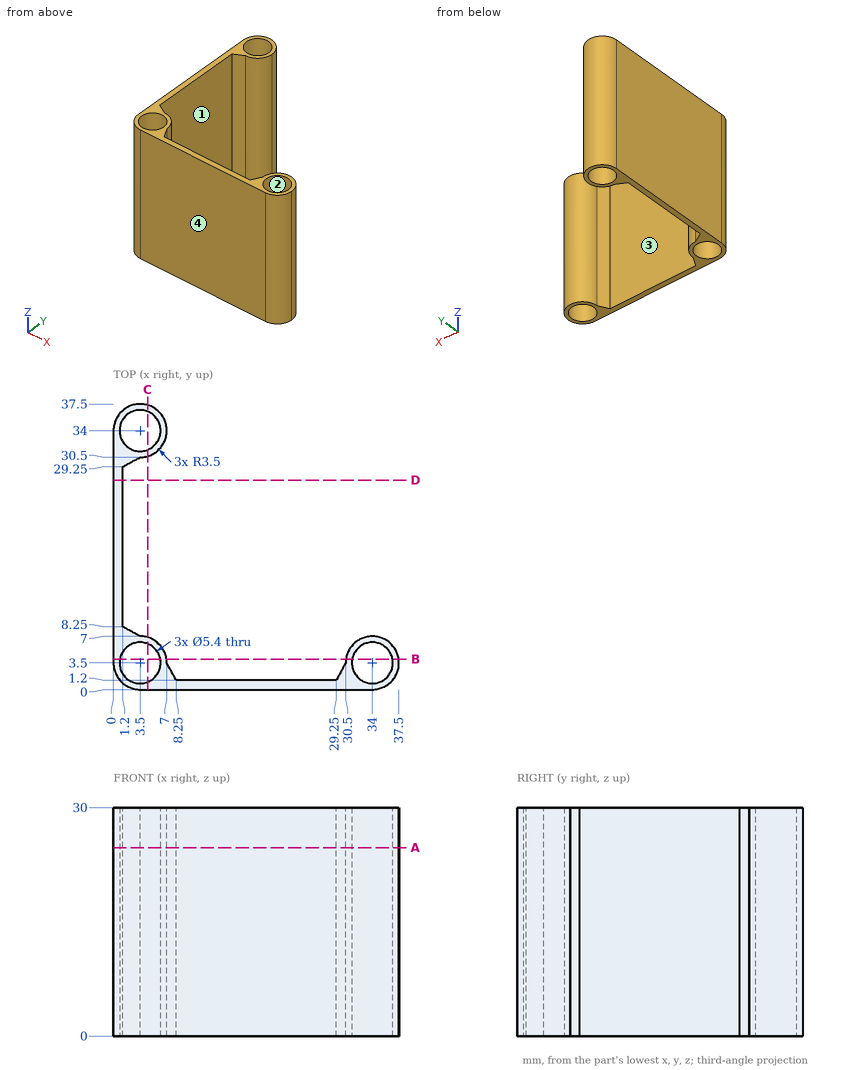
Could you check a few things on this drawing? It's one solid part, dimensions in mm from its lowest x, y, z. Coordinates: 2 decimals unless noted, no trailing zeros. Write each loop counter-clockwise with the first axis right and the second up, starting at its lowest first coordinate (ties: lowest second). Pieces come first, ordered by that corner, then holes. Notation, with made-up numbers: (33, 83.25) - (51, 83.25) arc R20 cw to (51, 89.25) - close; hole circle Ø1 at (-36, 7.25). An arc over 180 degrees is marked (long way). Return JSON: item names as keys, results as strings. Group by question number.
Item 1: If we section it at C-C (x = 4.5): Write out the boundary of the cut face in (y, z), then the cut area to 3 significant figures.
Item 2: If we section it at D-D (y = 27.5): Write out the boundary of the cut face in (x, z), then the cut area to 3 significant figures.
Item 3: If we section it at B-B (y = 4): Write out the boundary of the cut face in (x, z).
Item 4: I'm going to push flat-ended pins straight in: pin 1 Ø10.5 at (y, z) = (15.5, 18.5) entering from +X; pin 2 Ø2 at (x, z) = (27, 23.5) entering from +Y; pin 3 Ø17 at (x, z) = (14.5, 13) entering from +Y. Where does each tip first touch, or does it pass through?
Item 5: If we section it at A-A (z = 24.75): Write out the boundary of the cut face in (x, y), then the cut area to 3 significant figures.
Item 6: We'd pull the mould along Y, two halves only. Please class the marked faces 1, 2, 3 and 4: pulls with the +Y half, pulls with the -Y half, needs draft (parallel to the pull), parting line crosses it, or undercut.
Item 7: Please list where these lines run through material, in increasing order: probe 1 along X at (y, z) = (5, 3) (3 decimals); probe 2 along X at (y, z) = (18, 19.5); probe 3 along Y at (x, z) = (4, 18.5).
Return value:
{
 "1": {"outline": "(0, 0) - (0.99, 0) - (0.99, 30) - (0, 30) - close; (6.01, 0) - (6.85, 0) - (6.85, 30) - (6.01, 30) - close; (30.65, 0) - (31.49, 0) - (31.49, 30) - (30.65, 30) - close; (36.51, 0) - (37.35, 0) - (37.35, 30) - (36.51, 30) - close", "area": "106 mm^2"},
 "2": {"outline": "(0, 0) - (1.2, 0) - (1.2, 30) - (0, 30) - close", "area": "36.0 mm^2"},
 "3": {"outline": "(0, 0) - (0.85, 0) - (0.85, 30) - (0, 30) - close; (6.15, 0) - (6.96, 0) - (6.96, 30) - (6.15, 30) - close; (30.54, 0) - (31.35, 0) - (31.35, 30) - (30.54, 30) - close; (36.65, 0) - (37.46, 0) - (37.46, 30) - (36.65, 30) - close"},
 "4": {"pin 1": "stops at x = 1.2", "pin 2": "stops at y = 1.2", "pin 3": "stops at y = 36.45"},
 "5": {"outline": "(0, 3.5) arc R3.5 ccw to (3.5, 0) - (34, 0) arc R3.5 ccw (long way) to (30.5, 3.5) - (29.25, 1.2) - (8.25, 1.2) - (7, 3.5) arc R3.5 ccw to (3.5, 7) - (1.2, 8.25) - (1.2, 29.25) - (3.5, 30.5) arc R3.5 ccw (long way) to (0, 34) - close; hole circle Ø5.4 at (3.5, 3.5); hole circle Ø5.4 at (3.5, 34); hole circle Ø5.4 at (34, 3.5)", "area": "119 mm^2"},
 "6": {"face 1": "undercut", "face 2": "undercut", "face 3": "pulls with the +Y half", "face 4": "pulls with the -Y half"},
 "7": {"probe 1": "x = 0 to 1.255, 5.745 to 6.662, 30.838 to 31.755, 36.245 to 37.162", "probe 2": "x = 0 to 1.2", "probe 3": "y = 0 to 0.85, 6.15 to 6.96, 30.54 to 31.35, 36.65 to 37.46"}
}
